```python
from build123d import *

# Parameters (mm, degrees)
SKETCH1_W           = 145
SKETCH1_H           = 90
BOSS_EXTRUDE1_DEPTH = 1
SKETCH2_W           = 140
SKETCH2_H           = 85
SKETCH2_W_2         = 135
SKETCH2_H_2         = 80
BOSS_EXTRUDE2_DEPTH = 5
FILLET1_R           = 2.5


with BuildPart() as part:
    # Sketch1 → Boss-Extrude1 (new body)
    with BuildSketch(Plane(origin=(0, 0, 0), x_dir=(1, 0, 0), z_dir=(0, 1, 0))):
        Rectangle(SKETCH1_W, SKETCH1_H)
    extrude(amount=-BOSS_EXTRUDE1_DEPTH)

    # Sketch2 → Boss-Extrude2 (add)
    with BuildSketch(Plane.XZ.offset(1)):
        Rectangle(SKETCH2_W, SKETCH2_H)
        Rectangle(SKETCH2_W_2, SKETCH2_H_2, mode=Mode.SUBTRACT)
    extrude(amount=BOSS_EXTRUDE2_DEPTH)

    # Fillet1
    fillet1_edges = [part.edges().sort_by_distance(p)[0] for p in [
        (72.5, -0.5, 45),
        (-72.5, -0.5, 45),
        (-72.5, -0.5, -45),
        (72.5, -0.5, -45),
    ]]
    fillet(fillet1_edges, radius=FILLET1_R)


solid = part.part
```
CAD build for the part. Positions are in the model's coordinates, mm. A direction names the side the tool comes from. Round coordinates to 2 decimals unless told otherwise and drop trailing zeros. Order: outer loops, then holes, each group sorted by start corner. A loop starts at its lowest first (then second) coordinate and runs counter-clockwise, first axis right, second up. Notation, with made-up numbers: (18.25, 64) - (67.25, 64) arc R13 ccw to (67.25, 80) - close; hole circle Ø4 at (69, -30). An arc over 180 degrees is marked (long way). Use CSV: the item, a comma, the result in double quotes. Start each with the question number.
1) Tool access for faces 1 (the flat face through (-1, -3, 40)), 2 (the flat face through (-1, -3, 42.5)), 3 (the flat face through (-1, -3, -42.5)): list every direction of +Z, -Z, +X, -X, +Y, -Y with a clear straight run to the whole face (end or side of a thin tool).
2) Wall check: L1, parallel to Z at x = 66, y = -3.2; L2, parallel to X at y = -3.05, z = -29; L3, parallel to Y at x = -1, z = 28. Give the ranges that are in metal, low to high. Write a range as [from, to].
3) Saw through at B-B (z = 26). List the corners of the cut face in (x, y), and give its area (3 significant figures).
4) Two-plate mould, pull along X, no slides. Class faces 4 (the flat face through (-1, 0, -1)), 5 (the flat face through (-70, -3, -1)), 6 (the flat face through (-67.5, -3, -1)), 7 (the flat face through (70, -3, -1)): pulls with the +X half, pulls with the -X half, needs draft (parallel to the pull), parting line crosses it, or undercut.
5) Pin check, flat tips, straight feed: pin 1 Ø2.5 at (x, y) = (-0.5, -3) entering from +Z; pin 2 Ø1.5 at (x, y) = (15, -2) entering from -Z; pin 3 Ø8 at (x, z) = (-51.5, 9) entering from -Y. Stop position of each tip, or through.
6) Saw through at A-A (y = -4.05). List the corners of the cut face in (x, z).
7) Saw through at C-C (x = 0). List the corners of the cut face in (y, z).
Values follow:
1,face 1,"-Y"
1,face 2,"+Z, +X, -X, -Y"
1,face 3,"-Z, +X, -X, -Y"
2,L1,"z = [-42.5, -40], [40, 42.5]"
2,L2,"x = [-70, -67.5], [67.5, 70]"
2,L3,"y = [-1, 0]"
3,outline,"(-72.5, -1) - (-70, -1) - (-70, -6) - (-67.5, -6) - (-67.5, -1) - (67.5, -1) - (67.5, -6) - (70, -6) - (70, -1) - (72.5, -1) - (72.5, 0) - (-72.5, 0) - close"
3,area,"170 mm2"
4,face 4,"needs draft"
4,face 5,"pulls with the -X half"
4,face 6,"undercut"
4,face 7,"pulls with the +X half"
5,pin 1,"stops at z = 42.5"
5,pin 2,"stops at z = -42.5"
5,pin 3,"stops at y = -1"
6,outline,"(-70, -42.5) - (70, -42.5) - (70, 42.5) - (-70, 42.5) - close; hole (-67.5, -40) - (67.5, -40) - (67.5, 40) - (-67.5, 40) - close"
7,outline,"(-6, -42.5) - (-1, -42.5) - (-1, -45) - (0, -45) - (0, 45) - (-1, 45) - (-1, 42.5) - (-6, 42.5) - (-6, 40) - (-1, 40) - (-1, -40) - (-6, -40) - close"
